Read the model definition and answer for the solid it produces. Units are mm, in the model's axes. Coordinates: 2 decimals unless noted, no trailing zeros. Write each loop counter-clockwise with the first axis right and the second up, starting at its lowest first coordinate (ties: lowest second). Pieces come first, ordered by that corner, then holes.
(1) Section C-C on y = 0.6 is taken. Write down the section's boundary in (x, z).
(2) Section D-D on x = -2 is taken. Write down the section's boundary in (y, z), then the cut area to 3 significant figures.
(3) Section A-A on z = 6.5 is taken. Write down the section's boundary in (x, y).
(4) Find the intervals of material crossed by probe 1 along Z at (x, y) = (-29, 1.4); probe 2 along X at (y, z) = (3, -10); probe 3 along X at (y, z) = (0.7, 11.5), in increasing order.
(5) Section B-B on x = 29 is taken. Write down the section's boundary in (y, z).
(6) Given pin 1 (4 mm diameter, centred on x = -5, z = 1.5, fed in from +Y); pin 2 (0.9 mm diameter, centred on y = 1.5, z = 5.5, fed in from +X); pin 3 (1.9 mm diameter, centred on x = 29, z = -10.18, fed in from -Y); pin 4 (2 mm diameter, centred on y = 1, z = 11.5, fed in from -X), each flat-ended and moving along its own axis, determine where each tip first touches the part or whether it passes through.
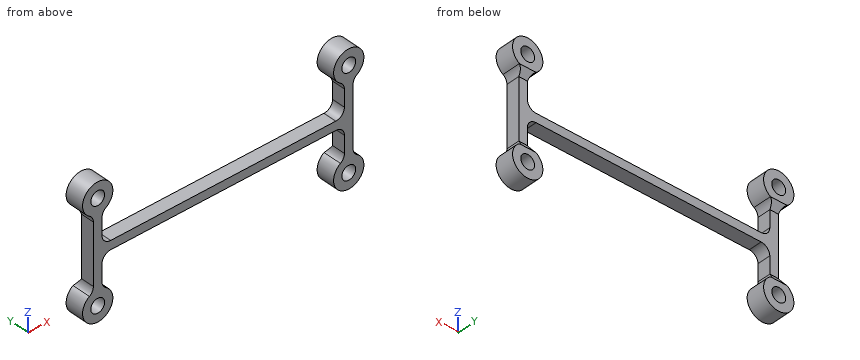
from build123d import *

# Parameters (mm, degrees)
BOSS_EXTRUDE1_DEPTH        = 4.25
F_3_2_3_2_DIAMETER_HOLE1_D = 3.2
CUT_EXTRUDE1_DEPTH         = 37.614339148
CUT_EXTRUDE1_DEPTH_BACK    = 37.614339148


with BuildPart() as part:
    # Sketch2 → Boss-Extrude1 (new body)
    with BuildSketch(Plane(origin=(0, 0, 0), x_dir=(1, 0, 0), z_dir=(0, 1, 0))):
        with BuildLine():
            Line((-26, -2.318619158), (26, -2.318619158))
            ThreePointArc((26, -2.318619158), (27.414213562, -2.904405596), (28, -4.318619158))
            Line((28, -4.318619158), (28, -8.208846929))
            ThreePointArc((28, -8.208846929), (27.758098146, -9.162309518), (27.090909091, -9.88512774))
            ThreePointArc((27.090909091, -9.88512774), (29, -16.318619158), (30.909090909, -9.88512774))
            ThreePointArc((30.909090909, -9.88512774), (30.241901854, -9.162309518), (30, -8.208846929))
            Line((30, -8.208846929), (30, 5.571608613))
            ThreePointArc((30, 5.571608613), (30.241901854, 6.525071203), (30.909090909, 7.247889424))
            ThreePointArc((30.909090909, 7.247889424), (29, 13.681380842), (27.090909091, 7.247889424))
            ThreePointArc((27.090909091, 7.247889424), (27.758098146, 6.525071203), (28, 5.571608613))
            Line((28, 5.571608613), (28, 1.681380842))
            ThreePointArc((28, 1.681380842), (27.414213562, 0.26716728), (26, -0.318619158))
            Line((26, -0.318619158), (-26, -0.318619158))
            ThreePointArc((-26, -0.318619158), (-27.414213562, 0.26716728), (-28, 1.681380842))
            Line((-28, 1.681380842), (-28, 5.571608613))
            ThreePointArc((-28, 5.571608613), (-27.758098146, 6.525071203), (-27.090909091, 7.247889424))
            ThreePointArc((-27.090909091, 7.247889424), (-29, 13.681380842), (-30.909090909, 7.247889424))
            ThreePointArc((-30.909090909, 7.247889424), (-30.241901854, 6.525071203), (-30, 5.571608613))
            Line((-30, 5.571608613), (-30, -8.208846929))
            ThreePointArc((-30, -8.208846929), (-30.241901854, -9.162309518), (-30.909090909, -9.88512774))
            ThreePointArc((-30.909090909, -9.88512774), (-29, -16.318619158), (-27.090909091, -9.88512774))
            ThreePointArc((-27.090909091, -9.88512774), (-27.758098146, -9.162309518), (-28, -8.208846929))
            Line((-28, -8.208846929), (-28, -4.318619158))
            ThreePointArc((-28, -4.318619158), (-27.414213562, -2.904405596), (-26, -2.318619158))
        make_face()
    extrude(amount=BOSS_EXTRUDE1_DEPTH)

    # Ø3.2 (3.2) Diameter Hole1 (through all)
    with Locations(Plane(origin=(0, 4.25, 0), x_dir=(1, 0, 0), z_dir=(0, 1, 0))):
        with Locations((-29, -12.818619158), (-29, 10.181380842), (29, 10.181380842), (29, -12.818619158)):
            Hole(F_3_2_3_2_DIAMETER_HOLE1_D / 2)

    # Sketch5 → Cut-Extrude1 (cut, two sides: drawn at the far end of the back side and taken through both)
    with BuildSketch(Plane(origin=(0, 0, 0), x_dir=(0, 0, -1), z_dir=(1, 0, 0)).offset(-CUT_EXTRUDE1_DEPTH_BACK)):
        Polygon((-8.208846929, 3.055472707), (5.571608613, 3.055472707), (7.247889424, 4.25), (-9.88512774, 4.25), align=None)
    extrude(amount=CUT_EXTRUDE1_DEPTH + CUT_EXTRUDE1_DEPTH_BACK, mode=Mode.SUBTRACT)


solid = part.part
Response:
1. outline: (-30.91, -7.25) arc R3.5 ccw (long way) to (-27.09, -7.25) arc R2 cw to (-28, -5.57) - (-28, -1.68) arc R2 cw to (-26, 0.32) - (26, 0.32) arc R2 cw to (28, -1.68) - (28, -5.57) arc R2 cw to (27.09, -7.25) arc R3.5 ccw (long way) to (30.91, -7.25) arc R2 cw to (30, -5.57) - (30, 8.21) arc R2 cw to (30.91, 9.89) arc R3.5 ccw (long way) to (27.09, 9.89) arc R2 cw to (28, 8.21) - (28, 4.32) arc R2 cw to (26, 2.32) - (-26, 2.32) arc R2 cw to (-28, 4.32) - (-28, 8.21) arc R2 cw to (-27.09, 9.89) arc R3.5 ccw (long way) to (-30.91, 9.89) arc R2 cw to (-30, 8.21) - (-30, -5.57) arc R2 cw to start; hole circle Ø3.2 at (-29, -10.18); hole circle Ø3.2 at (-29, 12.82); hole circle Ø3.2 at (29, -10.18); hole circle Ø3.2 at (29, 12.82)
2. outline: (0, 0.32) - (3.06, 0.32) - (3.06, 2.32) - (0, 2.32) - close
2. area: 6.11 mm2
3. outline: (-30, 0) - (-28, 0) - (-28, 3.06) - (-30, 3.06) - close; (28, 0) - (30, 0) - (30, 3.06) - (28, 3.06) - close
4. probe 1: z = -13.68 to -11.78, -8.58 to 11.22, 14.42 to 16.32
4. probe 2: x = -32.5 to -30.59, -27.41 to -25.5, 25.5 to 27.41, 30.59 to 32.5
4. probe 3: x = -32.24 to -29.91, -28.09 to -25.76, 25.76 to 28.09, 29.91 to 32.24
5. outline: (0, -13.68) - (4.25, -13.68) - (4.25, -11.78) - (0, -11.78) - close; (0, -8.58) - (4.25, -8.58) - (4.25, -7.25) - (3.06, -5.57) - (3.06, 8.21) - (4.25, 9.89) - (4.25, 11.22) - (0, 11.22) - close; (0, 14.42) - (4.25, 14.42) - (4.25, 16.32) - (0, 16.32) - close
6. pin 1: stops at y = 3.06
6. pin 2: stops at x = 30
6. pin 3: passes through
6. pin 4: stops at x = -32.49
